Autodesk Fusion 360 part; units mm, degrees
sketch "Sketch1" plane through (0, 0, 0) normal (0, 0, 1) x (1, 0, 0)
  line L0 (0, 0) -> (9.5, 0)
  line L1 (9.5, 0) -> (9.5, 25)
  line L2 (9.5, 25) -> (0, 25)
  line L3 (0, 25) -> (0, 0)
  line L4 (1.25, 25) -> (8.25, 25)
  line L5 (8.25, 25) -> (8.25, 0)
  line L6 (8.25, 0) -> (1.25, 0)
  line L7 (1.25, 0) -> (1.25, 25)
  line L8 (3, 0) -> (0, 6.4335)
  line L9 (3, 0) -> (6, 0) construction
  line L10 (6.5, 0) -> (9.5, 6.4335)
  dimension "d1" = 9.5
  dimension "d2" = 25
  dimension "d3" = 7
  dimension "d4" = 1.25
  dimension "d11" = 3
  dimension "d12" = 3
  dimension "d13" = 65
  dimension "d14" = 65
extrude "Extrude1" add sketch "Sketch1" along normal blind 2 contours L2 L3 L7 L8 | L0 L2 L4 L5 L6 L7 L8 L10 | L1 L2 L5 L10
extrude "Extrude2" add sketch "Sketch1" along normal blind 12 contours L0 L2 L4 L5 L6 L7 L8 L10
sketch "Sketch3" plane through (0, 0, 12) normal (0, 0, 1) x (-1, 0, 0)
  line L0 (-3, 0) -> (-6.5, 0)
  line L1 (-6.5, 0) -> (-8.25, -3.7529)
  line L2 (-8.25, -3.7529) -> (-8.25, -25)
  line L3 (-8.25, -25) -> (-1.25, -25)
  line L4 (-1.25, -25) -> (-1.25, -3.7529)
  line L5 (-1.25, -3.7529) -> (-3, 0)
  line L6 (-1.25, -35) -> (-8.25, -35)
  line L7 (-8.25, -35) -> (-8.25, 10)
  line L8 (-8.25, 10) -> (-1.25, 10)
  line L9 (-1.25, 10) -> (-1.25, -35)
  line L10 (-8.25, -35) -> (-1.25, -35)
  line L11 (-1.25, -35) -> (-1.25, -32)
  line L12 (-1.25, -32) -> (-8.25, -32)
  line L13 (-8.25, -32) -> (-8.25, -35)
  line L14 (-1.25, 10) -> (-8.25, 10)
  line L15 (-8.25, 10) -> (-8.25, 7)
  line L16 (-8.25, 7) -> (-1.25, 7)
  line L17 (-1.25, 7) -> (-1.25, 10)
  dimension "d25" = 10
  dimension "d26" = 10
  dimension "d27" = 3
  dimension "d28" = 3
extrude "Extrude3" add sketch "Sketch3" along normal blind 2.5
extrude "Extrude4" add sketch "Sketch3" against normal blind 2 contours L7 L8 L9 L14 L15 L16 L17 | L6 L7 L9 L10 L11 L12 L13
Read the model definition and answer for the solid it produces. Units are mm, in the model's axes. A direction names the side the tool comes from. Give positions to 0.01 mm unless a question says otherwise; leave off trailing zeros. Loops run counter-clockwise (first coordinate to the right, second up) from the corner with the lowest first, then second, coordinate; pieces in that order, holes last. Notation, with made-up numbers: (55, 52.25) -> (97, 52.25) arc R9 cw to (97, 64.25) -> close; hole circle Ø8 at (64, 6). An arc over 180 degrees is marked (long way). Answer as CSV lines item,"result".
Item 1: Find section B-B on x = 2.5. Give the vertices of the cut face in (y, z).
Returned:
outline,"(-10, 10) -> (-7, 10) -> (-7, 12) -> (1.07, 12) -> (1.07, 0) -> (25, 0) -> (25, 12) -> (32, 12) -> (32, 10) -> (35, 10) -> (35, 14.5) -> (-10, 14.5) -> close"
Item 2: Each of these flat-tipped pins is pushed along its axis until it touches: pin 1 (1.4 mm diameter, centred on x = 0.5, y = 17, fed in from +Z); pin 2 (3.5 mm diameter, centred on x = 4.5, y = 28.5, fed in from -Z); pin 3 (3.5 mm diameter, centred on x = 5, y = 34, fed in from -Z). Where does it stop, or does it pass through?
Returned:
pin 1,"stops at z = 2"
pin 2,"stops at z = 12"
pin 3,"stops at z = 10"
Item 3: For faces 1 (the face through (8.25, 12, 10)), 2 (the face through (5, 32, 11)), 3 (the face through (1.25, 13, 10)), 4 (the face through (5, -9, 10)), determine the directions among +Z, -Z, +X, -X, +Y, -Y from which every point of the face is accessible in a straight line to the end or side of a thin tool.
Returned:
face 1,"+Z, +X, +Y, -Y"
face 2,"-Z, +X, -X"
face 3,"+Z, -X, +Y, -Y"
face 4,"-Z, +X, -X, -Y"
Item 4: Find section D-D on z = 4.5. Give the vertices of the cut face in (x, y), plus the area to 3 significant figures.
Returned:
outline,"(1.25, 3.75) -> (3, 0) -> (6.5, 0) -> (8.25, 3.75) -> (8.25, 25) -> (1.25, 25) -> close"
area,"168 mm²"
Item 5: Determine the mould class of faces 5 (the face through (1, 15, 2)), 6 (the face through (5, -10, 12)), 7 (the face through (5, 28, 12)), 8 (the face through (5, 35, 12)) for opening direction Y: +Y half, -Y half, draft (parallel to the pull), parting line (faces both ways), or undercut.
Returned:
face 5,"draft"
face 6,"-Y half"
face 7,"undercut"
face 8,"+Y half"
Item 6: Find section C-C on y = 17. Give the vertices of the cut face in (x, z), plus the area to 4 significant figures.
Returned:
outline,"(0, 0) -> (9.5, 0) -> (9.5, 2) -> (8.25, 2) -> (8.25, 14.5) -> (1.25, 14.5) -> (1.25, 2) -> (0, 2) -> close"
area,"106.5 mm²"
Item 7: Find section A-A on z = 10.75. Give the vertices of the cut face in (x, y).
Returned:
outline,"(1.25, -10) -> (8.25, -10) -> (8.25, -7) -> (1.25, -7) -> close; (1.25, 3.75) -> (3, 0) -> (6.5, 0) -> (8.25, 3.75) -> (8.25, 25) -> (1.25, 25) -> close; (1.25, 32) -> (8.25, 32) -> (8.25, 35) -> (1.25, 35) -> close"
Item 8: Consider line 1 (Y direction, x = 4, z = 11.5); line 2 (Y direction, x = 5, z = 6.75); line 3 (X direction, y = 13.5, z = 2.75). Determine where each line is inside the solid, lowest interval first. Write a range as [from, to].
Returned:
line 1,"y = [-10, -7], [0, 25], [32, 35]"
line 2,"y = [0, 25]"
line 3,"x = [1.25, 8.25]"
